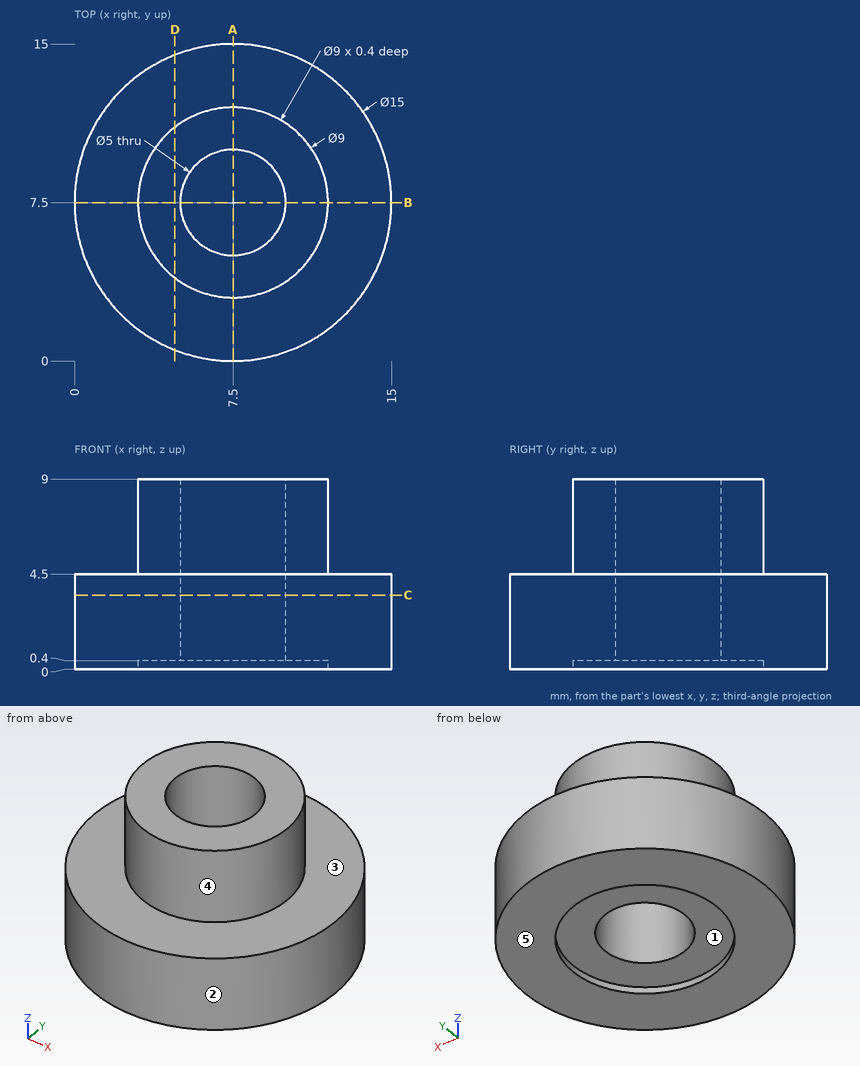
Verification items for this drawing (mm, ordinates from the low corner). A direction names the side the tool comes from. Round coordinates to 2 decimals unless told otherwise and drop trailing zeros. Loops run counter-clockwise (first coordinate to the right, second up) from the corner with the lowest first, then second, coordinate; pieces in that order, holes last. Notation, with made-up numbers: (8.25, 73) - (52.25, 73) arc R17 ccw to (52.25, 92) - close; hole circle Ø1 at (25.5, 61.5). An arc over 180 degrees is marked (long way). Answer as CSV lines item,"result". Start each with the question number.
Item 1: Set-up check for the marked faces 4 and 5: record each of +Z, -Z, +X, -X, +Y, -Y from which the full face is reachable in a straight line by a thin tool's end or side.
Item 2: Section check C-C (z = 3.5). Record the boundary of the cut face in (x, y).
Item 3: Scan lines: line 1 (Y direction, x = 7.5, z = 7.25); line 2 (Y direction, x = 7.5, z = 0.25); line 3 (Z direction, x = 3, y = 11.75). Record each from-to range of solid material in increasing order. Write a range as [from, to].
Item 4: Release check for a two-part mould opening along Y. For the marked faces 1, 2 and 3 record: +Y half, -Y half, draft (parallel to the pull), parting line (faces both ways), or undercut.
Item 5: Section check A-A (x = 7.5). Record the boundary of the cut face in (y, z).
Item 6: Section check D-D (x = 4.75). Record the boundary of the cut face in (y, z), and give its area (3 significant figures).
Item 7: Depth check by flat-ended pin: P1, Ø1.5, axis at x = 10, z = 6.5, coming from the -Y side; P2, Ø6, axis at x = 7.5, y = 7.5, coming from the +Z side; P3, Ø5, axis at y = 12.5, z = 2.5, coming from the +X side; P4, Ø1.5, axis at y = 11.5, z = 7.5, coming from the -X side. Enter the tip coordinate at first touch or a pass-through.
Report:
1,face 4,"+Z"
1,face 5,"-Z, +X, -X, +Y, -Y"
2,outline,"circle Ø15 at (7.5, 7.5); hole circle Ø5 at (7.5, 7.5)"
3,line 1,"y = [3, 5], [10, 12]"
3,line 2,"y = [0, 3], [12, 15]"
3,line 3,"z = [0, 4.5]"
4,face 1,"undercut"
4,face 2,"parting line"
4,face 3,"draft"
5,outline,"(0, 0) - (3, 0) - (3, 0.4) - (5, 0.4) - (5, 9) - (3, 9) - (3, 4.5) - (0, 4.5) - close; (10, 0.4) - (12, 0.4) - (12, 0) - (15, 0) - (15, 4.5) - (12, 4.5) - (12, 9) - (10, 9) - close"
6,outline,"(0.52, 0) - (3.94, 0) - (3.94, 0.4) - (11.06, 0.4) - (11.06, 0) - (14.48, 0) - (14.48, 4.5) - (11.06, 4.5) - (11.06, 9) - (3.94, 9) - (3.94, 4.5) - (0.52, 4.5) - close"
6,area,"92.0 mm2"
7,P1,"stops at y = 3.35"
7,P2,"stops at z = 9"
7,P3,"stops at x = 14.57"
7,P4,"stops at x = 4.39"
